Work out the finished part from the listing and answer in its coordinate system (mm). Face numbers are marked on the shaded views. A direction names the side the tool comes from. Round coordinates to 2 decimals unless told otherwise and drop trailing zeros. Loops run counter-clockwise (first coordinate to the right, second up) from the corner with the lowest first, then second, coordinate; pieces in that order, holes last.
```python
from build123d import *

# Parameters (mm, degrees)
SKETCH1_W               = 5.6
SKETCH1_H               = 40
BOSS_EXTRUDE1_DEPTH     = 4
SKETCH2_W               = 5.6
SKETCH2_H               = 2
BOSS_EXTRUDE2_DEPTH     = 4
SKETCH4_W               = 4
SKETCH4_H               = 4.2
BOSS_EXTRUDE3_DEPTH     = 1.8
MIRROR2_COPY_1_SKETCH_W = 4
MIRROR2_COPY_1_SKETCH_H = 4.2
MIRROR2_COPY_1_DEPTH    = 1.8
SKETCH8_W               = 4
SKETCH8_H               = 4.2
BOSS_EXTRUDE4_DEPTH     = 8
SKETCH9_W               = 17.2
SKETCH9_H               = 2.1
BOSS_EXTRUDE5_DEPTH     = 4
SKETCH10_W              = 4
SKETCH10_H              = 12.8
BOSS_EXTRUDE6_DEPTH     = 7.5
SKETCH11_R              = 1.5
CUT_EXTRUDE1_DEPTH      = 1


with BuildPart() as part:
    # Sketch1 → Boss-Extrude1 (new body)
    with BuildSketch(Plane.XY):
        Rectangle(SKETCH1_W, SKETCH1_H)
    extrude(amount=BOSS_EXTRUDE1_DEPTH)

    # Sketch2 → Boss-Extrude2 (add)
    with BuildSketch(Plane.XY.offset(4)):
        with Locations((0, -19)):
            Rectangle(SKETCH2_W, SKETCH2_H)
    extrude(amount=BOSS_EXTRUDE2_DEPTH)

    # Sketch4 → Boss-Extrude3 (add)
    with BuildSketch(Plane.ZY.offset(2.8)):
        with Locations((2, 9.6)):
            Rectangle(SKETCH4_W, SKETCH4_H)
    boss_extrude3 = extrude(amount=BOSS_EXTRUDE3_DEPTH)

    # Mirror1: Boss-Extrude3 across plane
    add(boss_extrude3.mirror(Plane.ZY))

    # Mirror2: Boss-Extrude3 across plane
    add(boss_extrude3.mirror(Plane(origin=(0, 1.1, 0), x_dir=(0, 0, 1), z_dir=(0, -1, 0))))

    # Mirror2 copy 1 sketch → Mirror2 copy 1 (add)
    with BuildSketch(Plane(origin=(2.8, 2.2, 0), x_dir=(0, 0, 1), z_dir=(1, 0, 0))):
        with Locations((2, 9.6)):
            Rectangle(MIRROR2_COPY_1_SKETCH_W, MIRROR2_COPY_1_SKETCH_H)
    extrude(amount=MIRROR2_COPY_1_DEPTH)

    # Sketch8 → Boss-Extrude4 (add)
    with BuildSketch(Plane.ZY.offset(4.6)):
        with Locations((2, 9.6)):
            Rectangle(SKETCH8_W, SKETCH8_H)
        with Locations((2, -7.4)):
            Rectangle(SKETCH8_W, SKETCH8_H)
    extrude(amount=BOSS_EXTRUDE4_DEPTH)

    # Sketch9 → Boss-Extrude5 (add)
    with BuildSketch(Plane.XY.offset(4)):
        with Locations((-4, 10.65)):
            Rectangle(SKETCH9_W, SKETCH9_H)
    extrude(amount=BOSS_EXTRUDE5_DEPTH)

    # Sketch10 → Boss-Extrude6 (add)
    with BuildSketch(Plane.ZY.offset(2.8)):
        with Locations((2, 1.1)):
            Rectangle(SKETCH10_W, SKETCH10_H)
    extrude(amount=BOSS_EXTRUDE6_DEPTH)

    # Sketch11 → Cut-Extrude1 (cut)
    with BuildSketch(Plane(origin=(0, 0, 0), x_dir=(-1, 0, 0), z_dir=(0, 0, -1))):
        with Locations((4.9, 1.1)):
            Circle(SKETCH11_R)
    extrude(amount=-CUT_EXTRUDE1_DEPTH, mode=Mode.SUBTRACT)


solid = part.part
```
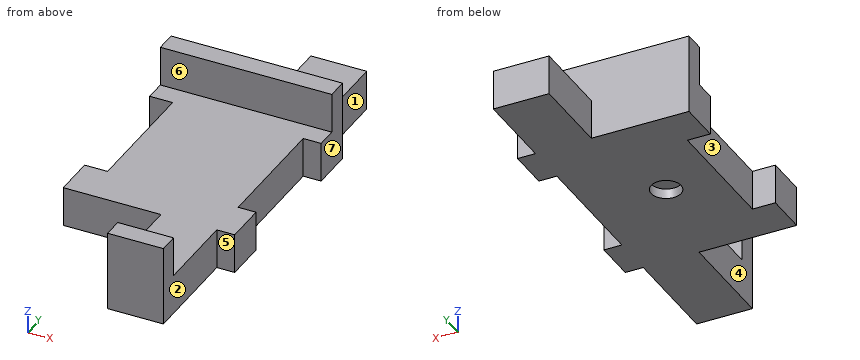
1. Find section B-B (z = 2.5). Write down the section's boundary in (x, y), then the cut area to 3 significant figures.
Answer key:
outline: (-12.6, -9.5) - (-2.8, -9.5) - (-2.8, -20) - (2.8, -20) - (2.8, -9.5) - (4.6, -9.5) - (4.6, -5.3) - (2.8, -5.3) - (2.8, 7.5) - (4.6, 7.5) - (4.6, 11.7) - (2.8, 11.7) - (2.8, 20) - (-2.8, 20) - (-2.8, 11.7) - (-12.6, 11.7) - (-12.6, 7.5) - (-10.3, 7.5) - (-10.3, -5.3) - (-12.6, -5.3) - close
area: 417 mm2
2. Consider probe 1 along Y at (x, z) = (-4.9, 0.6); probe 2 along Y at (x, z) = (0, 4.75); probe 3 along Z at (x, y) = (1, -11.5). Determine where each line is inside the solid, lowest interval first.
Answer key:
probe 1: y = -9.5 to -0.4, 2.6 to 11.7
probe 2: y = -20 to -18, 9.6 to 11.7
probe 3: z = 0 to 4
3. Determine the mould class of the marked faces 5, 6 and 7 for opening direction Y: +Y half, -Y half, draft (parallel to the pull), parting line (faces both ways), or undercut.
Answer key:
face 5: -Y half
face 6: undercut
face 7: draft
4. Find section C-C (x = -4.9). Write down the section's boundary in (y, z), then the cut area to 3 significant figures.
Answer key:
outline: (-9.5, 0) - (-0.4, 0) - (-0.4, 1) - (2.6, 1) - (2.6, 0) - (11.7, 0) - (11.7, 8) - (9.6, 8) - (9.6, 4) - (-9.5, 4) - close
area: 90.2 mm2
5. Find section A-A (z = 7.25). Write down the section's boundary in (x, y), then the cut area to 3 significant figures.
Answer key:
outline: (-12.6, 9.6) - (4.6, 9.6) - (4.6, 11.7) - (-12.6, 11.7) - close; (-2.8, -20) - (2.8, -20) - (2.8, -18) - (-2.8, -18) - close
area: 47.3 mm2
6. Find section D-D (y = 1.1). Write down the section's boundary in (x, z).
Answer key:
outline: (-10.3, 0) - (-6.4, 0) - (-6.4, 1) - (-3.4, 1) - (-3.4, 0) - (2.8, 0) - (2.8, 4) - (-10.3, 4) - close
7. Given pin 1 (4.5 mm diameter, centred on x = -5.5, z = 5.5, fed in from -Y); pin 2 (2.5 mm diameter, centred on y = -12.5, z = 3.5, fed in from -X); pin 3 (2 mm diameter, centred on y = 3, z = 1.5, fed in from -X), each flat-ended and moving along its own axis, determine where each tip first touches the part or whether it passes through.
Answer key:
pin 1: stops at y = -9.5
pin 2: stops at x = -2.8
pin 3: stops at x = -10.3
8. Which of the six approach directions +Z, -Z, +X, -X, +Y, -Y give full straight-line access (tool end or side, diameter ignored) to the marked faces 1, 2, 3 and 4?
Answer key:
face 1: +Z, -Z, +X, +Y
face 2: +Z, -Z, +X, -Y
face 3: +Z, -Z, -X
face 4: +Z, -Z, -X, -Y
